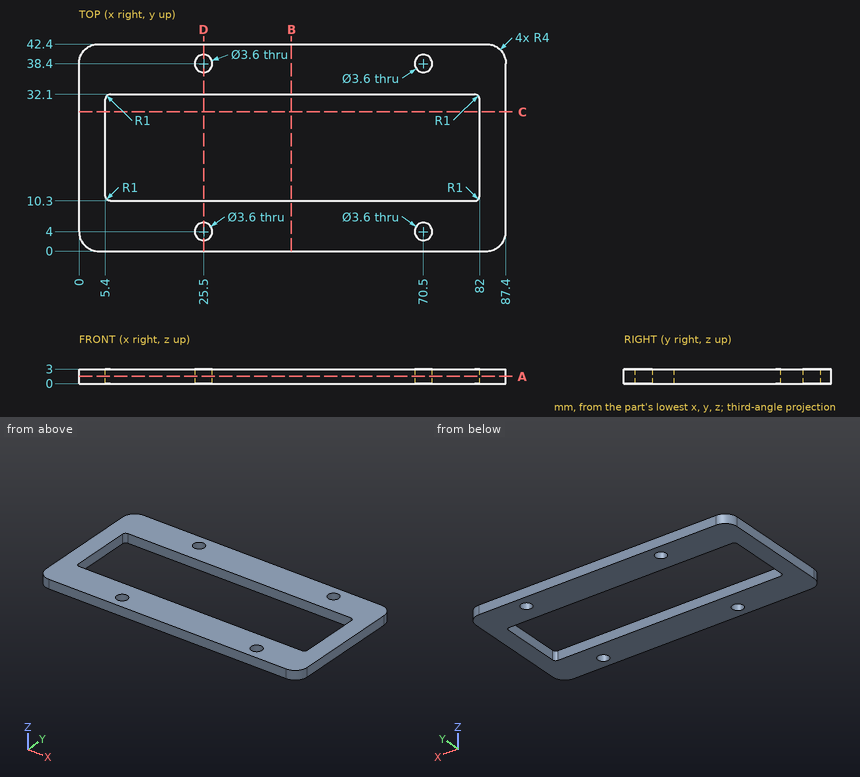
Input: dimensioned drawing with shaded views. Units: mm. Origin: part minimum x, y, z. Give positions to 0.01 mm unless a question says otherwise; leave off trailing zeros. Loops run counter-clockwise (first coordinate to the right, second up) from the corner with the lowest first, then second, coordinate; pieces in that order, holes last. Notation, with made-up numbers: M 63.25,26 L 94.25,26 A22 ccw 94.25,49 Z; hole C 69.5,60 d2. An arc over 180 degrees is marked long. Put each result on its own line as item: value.
1) Cut plane C-C, the plane y = 28.5. Return the cut outline in (x, z).
Computed values:
outline: M 0,0 L 5.4,0 L 5.4,3 L 0,3 Z; M 82,0 L 87.4,0 L 87.4,3 L 82,3 Z
2) Material intervals for L1, parallel to Y at x = 70.5, z = 0.9; L2, parallel to Y at x = 57, z = 1.75; L3, parallel to X at y = 12.5, z = 2, sorted ascending. Write a range as from..to.
Computed values:
L1: y = 0..2.2, 5.8..10.3, 32.1..36.6, 40.2..42.4
L2: y = 0..10.3, 32.1..42.4
L3: x = 0..5.4, 82..87.4
3) Cut plane D-D, the plane x = 25.5. Return the cut outline in (y, z).
Computed values:
outline: M 0,0 L 2.2,0 L 2.2,3 L 0,3 Z; M 5.8,0 L 10.3,0 L 10.3,3 L 5.8,3 Z; M 32.1,0 L 36.6,0 L 36.6,3 L 32.1,3 Z; M 40.2,0 L 42.4,0 L 42.4,3 L 40.2,3 Z
4) Cut plane A-A, the plane z = 1.5. Return the cut outline in (x, y).
Computed values:
outline: M 0,4 A4 ccw 4,0 L 83.4,0 A4 ccw 87.4,4 L 87.4,38.4 A4 ccw 83.4,42.4 L 4,42.4 A4 ccw 0,38.4 Z; hole M 5.4,11.3 A1 ccw 6.4,10.3 L 81,10.3 A1 ccw 82,11.3 L 82,31.1 A1 ccw 81,32.1 L 6.4,32.1 A1 ccw 5.4,31.1 Z; hole C 25.5,4 d3.6; hole C 25.5,38.4 d3.6; hole C 70.5,4 d3.6; hole C 70.5,38.4 d3.6
5) Cut plane B-B, the plane x = 43.5. Return the cut outline in (y, z).
Computed values:
outline: M 0,0 L 10.3,0 L 10.3,3 L 0,3 Z; M 32.1,0 L 42.4,0 L 42.4,3 L 32.1,3 Z
